Check sheet for the modelled part. Datum: model origin and axes. Units: mm. Face numbers are marked on the shaded views. Round coordinates to 2 decimals unless told otherwise and drop trailing zeros. Write each loop counter-clockwise with the first axis right and the second up, starting at its lowest first coordinate (ties: lowest second). Pieces come first, ordered by that corner, then holes. Notation, with made-up numbers: M 47.25,63.5 L 90.25,63.5 A28 ccw 90.25,93.5 Z; hole C 77,14.25 d5. An arc over 180 degrees is marked long. Answer in a Markdown table with one row per item.
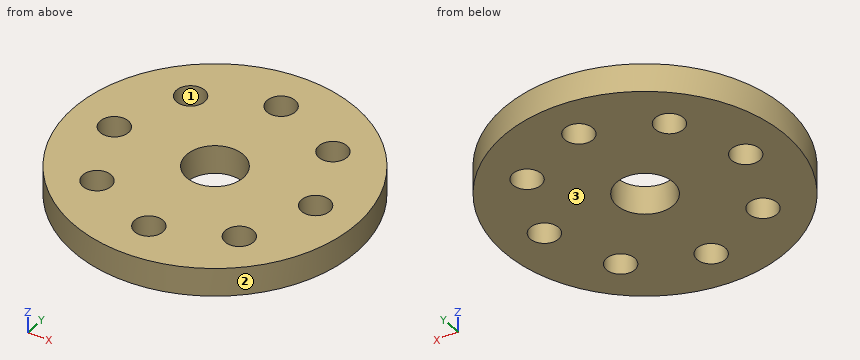
```python
from build123d import *

# Parameters (mm, degrees)
F0_R     = 63.5
F0_R_2   = 6.35
F0_R_3   = 12.7
F1_DEPTH = 12.7


with BuildPart() as f1:
    # F0 (on Top) → F1 (new body)
    with BuildSketch(Plane.XY):
        Circle(F0_R)
        with Locations((-31.430896, -31.430896)):
            Circle(F0_R_2, mode=Mode.SUBTRACT)
        with Locations((0, -44.45)):
            Circle(F0_R_2, mode=Mode.SUBTRACT)
        with Locations((31.430896, -31.430896)):
            Circle(F0_R_2, mode=Mode.SUBTRACT)
        with Locations((-44.45, 0)):
            Circle(F0_R_2, mode=Mode.SUBTRACT)
        with Locations((-31.430896, 31.430896)):
            Circle(F0_R_2, mode=Mode.SUBTRACT)
        Circle(F0_R_3, mode=Mode.SUBTRACT)
        with Locations((31.430896, 31.430896)):
            Circle(F0_R_2, mode=Mode.SUBTRACT)
        with Locations((44.45, 0)):
            Circle(F0_R_2, mode=Mode.SUBTRACT)
        with Locations((0, 44.45)):
            Circle(F0_R_2, mode=Mode.SUBTRACT)
    extrude(amount=-F1_DEPTH)


solid = f1.part
```
1. Go/stop test with flat-tipped pins: pin 1 (1 mm diameter, centred on y = -26, z = -5, fed in from +X); pin 2 (3 mm diameter, centred on x = 37, z = -9, fed in from -Y); pin 3 (5 mm diameter, centred on y = 47, z = -3, fed in from +X). Record where each tip stops, or that it passes through.
Found:
| item | result |
|---|---|
| pin 1 | stops at x = 58.15 |
| pin 2 | stops at y = -52.65 |
| pin 3 | stops at x = 45.3 |
2. Scan lines: L1, parallel to X at y = 0.5, z = -5.5; L2, parallel to Y at x = 0, z = -6.5; L3, parallel to Y at x = -27.5, z = -8.75. Record each from-to range of solid material in increasing order.
Found:
| item | result |
|---|---|
| L1 | x = -63.5 to -50.78, -38.12 to -12.69, 12.69 to 38.12, 50.78 to 63.5 |
| L2 | y = -63.5 to -50.8, -38.1 to -12.7, 12.7 to 38.1, 50.8 to 63.5 |
| L3 | y = -57.24 to -36.42, -26.44 to 26.44, 36.42 to 57.24 |
3. Section check A-A, the plane x = 0. Record the cut outline in (y, z), and give its area (3 significant figures).
Found:
| item | result |
|---|---|
| outline | M -63.5,-12.7 L -50.8,-12.7 L -50.8,0 L -63.5,0 Z; M -38.1,-12.7 L -12.7,-12.7 L -12.7,0 L -38.1,0 Z; M 12.7,-12.7 L 38.1,-12.7 L 38.1,0 L 12.7,0 Z; M 50.8,-12.7 L 63.5,-12.7 L 63.5,0 L 50.8,0 Z |
| area | 968 mm2 |
4. Section check C-C, the plane z = -8. Count the separate pieces of the cut face and the enclosed holes in it, and give its area (3 significant figures).
Found:
| item | result |
|---|---|
| separate pieces | 1 |
| enclosed holes | 9 |
| area | 11,100 mm2 |
5. Section check D-D, the plane x = 30. Record the cut outline in (y, z), and give its area (3 significant figures).
Found:
| item | result |
|---|---|
| outline | M -55.97,-12.7 L -37.62,-12.7 L -37.62,0 L -55.97,0 Z; M -25.24,-12.7 L 25.24,-12.7 L 25.24,0 L -25.24,0 Z; M 37.62,-12.7 L 55.97,-12.7 L 55.97,0 L 37.62,0 Z |
| area | 1,110 mm2 |
6. Draft check along X on the marked faces 1, 2 and 3. Enter one of: +X half, -X half, draft (parallel to the pull), parting line (faces both ways), or undercut.
Found:
| item | result |
|---|---|
| face 1 | undercut |
| face 2 | parting line |
| face 3 | draft |
